Work out the finished part from the listing and answer in its coordinate system (mm). Face numbers are marked on the shaded views. A direction names the side the tool comes from. Coordinates: 2 decimals unless noted, no trailing zeros. Loops run counter-clockwise (first coordinate to the right, second up) from the corner with the lowest first, then second, coordinate; pieces in that order, holes last. Notation, with made-up numbers: (-8.75, 51.5) -> (-1.75, 51.5) arc R20 cw to (-1.75, 60.5) -> close; hole circle Ø2 at (79.25, 61.5). An arc over 180 degrees is marked (long way). Answer as CSV lines item,"result".
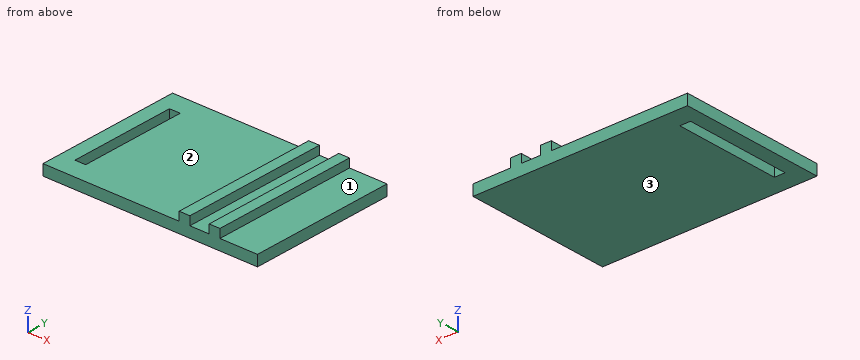
Autodesk Inventor part; units mm, degrees
ref_plane "YZ Plane" through (0, 0, 0) normal (1, 0, 0) x (0, 1, 0)
ref_plane "XZ Plane" through (0, 0, 0) normal (0, 1, 0) x (-1, 0, 0)
ref_plane "XY Plane" through (0, 0, 0) normal (0, 0, 1) x (1, 0, 0)
sketch "Sketch1" plane through (0, 0, 0) normal (0, 0, 1) x (1, 0, 0)
  line L0 (0, 0) -> (20, 0)
  line L1 (20, 0) -> (20, 13.7)
  line L2 (20, 13.7) -> (0, 13.7)
  line L3 (0, 13.7) -> (0, 0)
  dimension "d0" = 20
  dimension "d1" = 13.7
extrude "Extrusion1" add sketch "Sketch1" along normal blind 1
sketch "Sketch2" plane through (0, 0, 1) normal (0, 0, 1) x (1, 0, 0)
  line L0 (0, 0) -> (20, 0)
  line L1 (20, 13.7) -> (0, 13.7)
  line L2 (13.7, 13.7) -> (12.7, 13.7)
  line L3 (12.7, 13.7) -> (12.7, 0)
  line L4 (12.7, 0) -> (13.7, 0)
  line L5 (13.7, 0) -> (13.7, 13.7)
  line L6 (15.5, 13.7) -> (16.5, 13.7)
  line L7 (16.5, 13.7) -> (16.5, 0)
  line L8 (16.5, 0) -> (15.5, 0)
  line L9 (15.5, 0) -> (15.5, 13.7)
  dimension "d4" = 1
  dimension "d5" = 1
  dimension "d6" = 1.8
  dimension "d9" = 3.5
extrude "Extrusion2" add sketch "Sketch2" along normal blind 0.8 contours L3 L1 L5 L0 | L9 L1 L7 L0
sketch "Sketch3" plane through (0, 0, 1) normal (0, 0, 1) x (1, 0, 0)
  line L0 (2.3449, 1.85) -> (1.3449, 1.85)
  line L1 (1.3449, 1.85) -> (1.3449, 11.85)
  line L2 (1.3449, 11.85) -> (2.3449, 11.85)
  line L3 (2.3449, 11.85) -> (2.3449, 1.85)
  line L4 (12.7, 13.7) -> (0, 13.7)
  line L5 (0, 0) -> (12.7, 0)
  dimension "d10" = 1
  dimension "d11" = 10
  dimension "d14" = 1.85
  dimension "d15" = 1.85
extrude "Extrusion3" cut sketch "Sketch3" against normal blind 10
properties part number "Zijkant 4"
(1) A cutting plane is placed at A-A, the plane y = 11.25. Write down the section's boundary in (x, z), and give its area (3 significant figures).
Computed values:
outline,"(0, 0) -> (1.34, 0) -> (1.34, 1) -> (0, 1) -> close; (2.34, 0) -> (20, 0) -> (20, 1) -> (16.5, 1) -> (16.5, 1.8) -> (15.5, 1.8) -> (15.5, 1) -> (13.7, 1) -> (13.7, 1.8) -> (12.7, 1.8) -> (12.7, 1) -> (2.34, 1) -> close"
area,"20.6 mm2"
(2) A cutting plane is placed at D-D, the plane x = 9. Write down the section's boundary in (y, z), and give its area (3 significant figures).
Computed values:
outline,"(0, 0) -> (13.7, 0) -> (13.7, 1) -> (0, 1) -> close"
area,"13.7 mm2"
(3) Flat-ended cylindrical pins translate along their axes: pin 1 Ø0.9 at (y, z) = (9.5, 1.5) entering from +X; pin 2 Ø4 at (x, y) = (3, 4) entering from +Z; pin 3 Ø0.6 at (y, z) = (4, 1.5) entering from -X. Find the tip coordinate at first contact, or state that the pin passes through.
Computed values:
pin 1,"x = 16.5"
pin 2,"z = 1"
pin 3,"x = 12.7"
(4) A cutting plane is placed at B-B, the plane z = 0.8. Write down the section's boundary in (x, y).
Computed values:
outline,"(0, 0) -> (20, 0) -> (20, 13.7) -> (0, 13.7) -> close; hole (1.34, 1.85) -> (2.34, 1.85) -> (2.34, 11.85) -> (1.34, 11.85) -> close"
(5) Which of the six approach directions +Z, -Z, +X, -X, +Y, -Y give full straight-line access (tool end or side, diameter ignored) to the marked faces 1, 2 and 3?
Computed values:
face 1,"+Z, +X, +Y, -Y"
face 2,"+Z, -X, +Y, -Y"
face 3,"-Z, +X, -X, +Y, -Y"
(6) Consider line 1 along X through (y, z) = (7, 0.1); line 2 along X through (y, z) = (1.75, 1.4); line 3 along Z through (x, y) = (7.5, 8.75). Determine where each line is inside the solid, lowest interval first.
Computed values:
line 1,"0 to 1.34, 2.34 to 20"
line 2,"12.7 to 13.7, 15.5 to 16.5"
line 3,"0 to 1"
(7) A cutting plane is placed at C-C, the plane y = 1.5. Write down the section's boundary in (x, z), and give its area (3 significant figures).
Computed values:
outline,"(0, 0) -> (20, 0) -> (20, 1) -> (16.5, 1) -> (16.5, 1.8) -> (15.5, 1.8) -> (15.5, 1) -> (13.7, 1) -> (13.7, 1.8) -> (12.7, 1.8) -> (12.7, 1) -> (0, 1) -> close"
area,"21.6 mm2"
